```python
from build123d import *

# Parameters (mm, degrees)
BOSS_EXTRUDE1_DEPTH = 1
SKETCH2_R           = 0.65
BOSS_EXTRUDE2_DEPTH = 5
SKETCH3_R           = 0.65
BOSS_EXTRUDE3_DEPTH = 5


with BuildPart() as part:
    # Sketch1 → Boss-Extrude1 (new, symmetric)
    with BuildSketch(Plane(origin=(0, 0, 0), x_dir=(0, 0, -1), z_dir=(1, 0, 0))):
        with BuildLine():
            Line((16.5, 1), (-9.5, 1))
            ThreePointArc((-9.5, 1), (-12.917652634, 2.648551595), (-16.5, 1.397608254))
            ThreePointArc((-16.5, 1.397608254), (-16.996560928, 0.198804127), (-16.5, -1))
            ThreePointArc((-16.5, -1), (-13, 0.449747468), (-9.5, -1))
            Line((-9.5, -1), (16.5, -1))
            ThreePointArc((16.5, -1), (17.5, 0), (16.5, 1))
        make_face()
    extrude(amount=BOSS_EXTRUDE1_DEPTH, both=True)

    # Sketch2 → Boss-Extrude2 (add)
    with BuildSketch(Plane(origin=(0, 0, 0), x_dir=(0, 0, -1), z_dir=(1, 0, 0))):
        with Locations((-16.5, 0)):
            Circle(SKETCH2_R)
    extrude(amount=-BOSS_EXTRUDE2_DEPTH)

    # Sketch3 → Boss-Extrude3 (add)
    with BuildSketch(Plane(origin=(0, 0, 0), x_dir=(0, 0, -1), z_dir=(1, 0, 0))):
        with Locations((16.5, 0)):
            Circle(SKETCH3_R)
    extrude(amount=-BOSS_EXTRUDE3_DEPTH)


solid = part.part
```
Source: CAD feature listing. Evaluate the final solid. Frame: model axes, mm. A direction names the side the tool comes from. Round coordinates to 2 decimals unless told otherwise and drop trailing zeros. Write each loop counter-clockwise with the first axis right and the second up, starting at its lowest first coordinate (ties: lowest second). Pieces come first, ordered by that corner, then holes. Notation, with made-up numbers: M 73.5,-2.75 L 132.5,-2.75 A25 ccw 132.5,14.25 Z; hole C 28.25,-8 d3. An arc over 180 degrees is marked long. Answer as a JSON object with one key per item and string values. Group by question number.
(1) Section query D-D on y = 2.1. Output: boundary loops of the cut face in (x, z).
(2) Section query A-A on y = 0. Output: boundary loops of the cut face in (x, z), then the cut area to 3 significant figures.
(3) First-contact query: pin 1 (2 mm diameter, centred on x = 0.5, z = -3.5, fed in from +Y); pin 2 (1 mm diameter, centred on y = 1.5, z = 9.5, fed in from -X). Flat tips, straight axial feed; report the tip coordinate or a pass-through.
(4) Section query B-B on x = -1.6. Output: boundary loops of the cut face in (y, z).
(5) Mould query, pull axis Z, two halves, no side actions, for faces 4 (the cylindrical face through (0.236, 0.217, 16.996)), 5 (the cylindrical face through (-3.02, 0.03, 17.15)), 6 (the flat face through (1, 0, 0)), 7 (the cylindrical face through (0.014, 2.645, 12.863)). Classes: +Z half, -Z half, draft (parallel to the pull), parting line (faces both ways), or undercut.
(6) Section query C-C on z = -4. Output: boundary loops of the cut face in (x, y), then the cut area to 3 significant figures.
(7) Reachability of faces 1 (the cylindrical face through (-2.97, 0.03, -15.85)), 2 (the cylindrical face through (0, 0, -17.5)), 3 (the flat face through (0, 1, -4)) from +Z, -Z, +X, -X, +Y, -Y: full face, straight path, thin tool, end or side. Return the list, or none.
(8) Ray query, line 1 (X direction, y = 0.8, z = 4); line 2 (Z direction, x = -2.15, y = 0.3). Return the intervals inside material, ascending. Write a range as [from, to].
Computed values:
{
 "1": {"outline": "M -1,10.92 L 1,10.92 L 1,15.48 L -1,15.48 Z"},
 "2": {"outline": "M -5,-17.15 L -1,-17.15 L -1,-17.5 L 1,-17.5 L 1,10.94 L -1,10.94 L -1,-15.85 L -5,-15.85 Z; M -5,15.85 L -1,15.85 L -1,15.06 L 1,15.06 L 1,16.98 L 0,16.98 L 0,17.15 L -5,17.15 Z", "area": "71.3 mm^2"},
 "3": {"pin 1": "y = 1", "pin 2": "x = -1"},
 "4": {"outline": "C 0,-16.5 d1.3; C 0,16.5 d1.3"},
 "5": {"face 4": "+Z half", "face 5": "undercut", "face 6": "draft", "face 7": "parting line"},
 "6": {"outline": "M -1,-1 L 1,-1 L 1,1 L -1,1 Z", "area": "4.00 mm^2"},
 "7": {"face 1": "-X", "face 2": "-Z, +X, -X", "face 3": "-Z, +X, -X, +Y"},
 "8": {"line 1": "[-1, 1]", "line 2": "[-17.08, -15.92], [15.92, 17.08]"}
}
